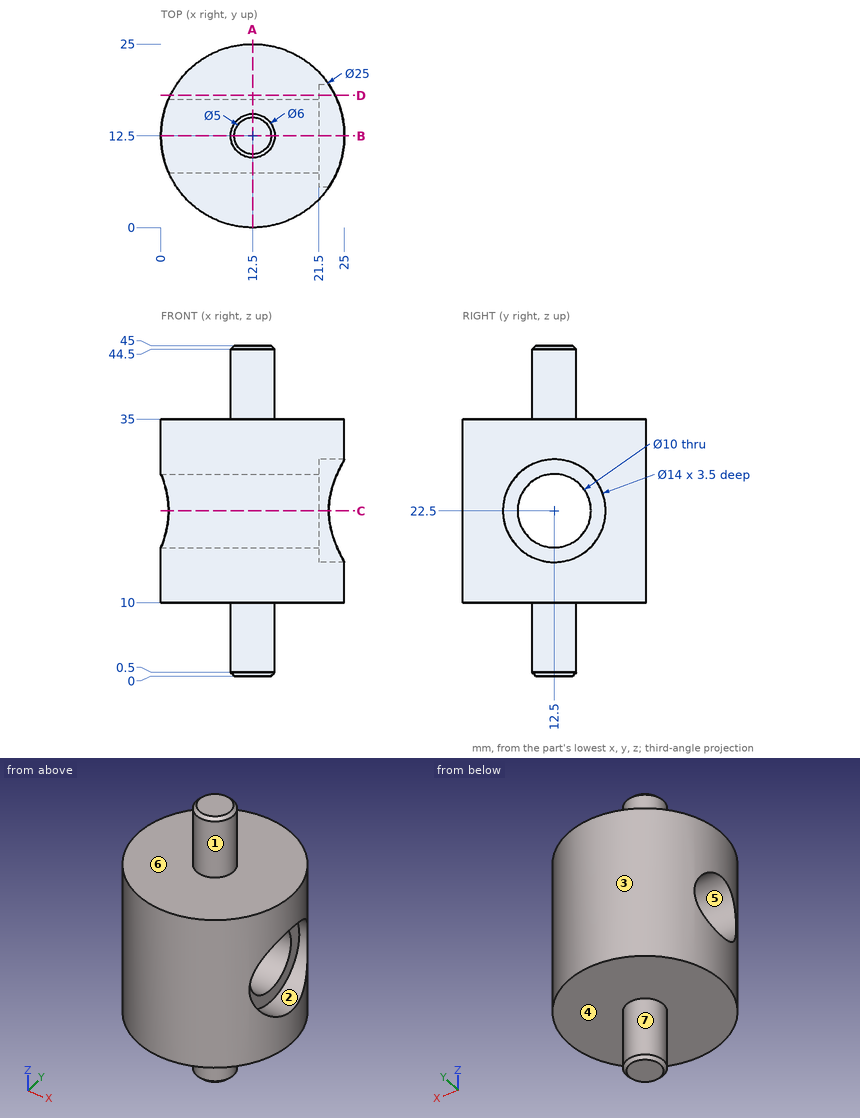
Design review of the part shown in the three views and the two pictorial views. Dimensions are in mm from the part's minimum x, y and z. A direction names the side the tool comes from. Give positions to 0.01 mm unless a question says otherwise; leave off trailing zeros. Loops run counter-clockwise (first coordinate to the right, second up) from the corner with the lowest first, then second, coordinate; pieces in that order, holes last. Notation, with made-up numbers: (-38, 78) - (-24, 78) arc R22 ccw to (-24, 102) - close; hole circle Ø2 at (-33, 10). An arc over 180 degrees is marked (long way). Write item = value, one per line.
1) Take a section at B-B on y = 12.5. State the section outline as (x, z) points, and give its area (4 significant figures).
Result sheet:
outline = (0, 10) - (9.5, 10) - (9.5, 0.5) - (10, 0) - (15, 0) - (15.5, 0.5) - (15.5, 10) - (25, 10) - (25, 15.5) - (21.5, 15.5) - (21.5, 17.5) - (0, 17.5) - close; (0, 27.5) - (21.5, 27.5) - (21.5, 29.5) - (25, 29.5) - (25, 35) - (15.5, 35) - (15.5, 44.5) - (15, 45) - (10, 45) - (9.5, 44.5) - (9.5, 35) - (0, 35) - close
area = 480.5 mm2
2) Take a section at C-C on z = 22.5. State the section outline as (x, y) points.
Result sheet:
outline = (1.04, 7.5) arc R12.5 ccw to (22.86, 5.5) - (21.5, 5.5) - (21.5, 7.5) - close; (1.04, 17.5) - (21.5, 17.5) - (21.5, 19.5) - (22.86, 19.5) arc R12.5 ccw to start
3) To check wall thickness, follow line 1 (Z direction, x = 7.75, y = 12.5); line 2 (Z direction, x = 11.25, y = 12.5); line 3 (Z direction, x = 6, y = 20.5). State the ranges of each line that lie inside material, in increasing order.
Result sheet:
line_1 = 10 to 17.5, 27.5 to 35
line_2 = 0 to 17.5, 27.5 to 45
line_3 = 10 to 35
4) Clearance check with flat-ended pins moving along their axes: pin 1 Ø4 at (x, y) = (18.5, 14) entering from -Z; pin 2 Ø11.5 at (y, z) = (12.5, 22.5) entering from -X; pin 3 Ø5 at (x, y) = (22.5, 22) entering from +Z; pin 4 Ø4 at (y, z) = (4, 13) entering from -X. State where each tip first meets the part, or that it passes through.
Result sheet:
pin_1 = 10
pin_2 = 0
pin_3 = 35
pin_4 = 1.82
5) Take a section at D-D on y = 18. State the section outline as (x, z) points, and give its area (3 significant figures).
Result sheet:
outline = (1.28, 10) - (23.72, 10) - (23.72, 18.17) - (21.5, 18.17) - (21.5, 26.83) - (23.72, 26.83) - (23.72, 35) - (1.28, 35) - close
area = 542 mm2
6) Take a section at A-A on x = 12.5. State the section outline as (y, z) points.
Result sheet:
outline = (0, 10) - (9.5, 10) - (9.5, 0.5) - (10, 0) - (15, 0) - (15.5, 0.5) - (15.5, 10) - (25, 10) - (25, 35) - (15.5, 35) - (15.5, 44.5) - (15, 45) - (10, 45) - (9.5, 44.5) - (9.5, 35) - (0, 35) - close; hole circle Ø10 at (12.5, 22.5)
7) Draft analysis for pull direction Z (two halves, no side actions). For the marked faces 4, 5, 6 and 7, state which applies: +Z half, -Z half, draft (parallel to the pull), parting line (faces both ways), or undercut.
Result sheet:
face_4 = -Z half
face_5 = undercut
face_6 = +Z half
face_7 = draft
8) Tool access review of the marked faces 1, 2 and 3: name each direction out of +Z, -Z, +X, -X, +Y, -Y from which nothing blocks a thin tool from reaching the whole face with its end or side.
Result sheet:
face_1 = +Z
face_2 = +X
face_3 = +Z, -Z
